Read the model definition and answer for the solid it produces. Units are mm, in the model's axes. Face numbers are marked on the shaded views. Coordinates: 2 decimals unless noted, no trailing zeros. Order: outer loops, then holes, each group sorted by start corner. A loop starts at its lowest first (then second) coordinate and runs counter-clockwise, first axis right, second up. Notation, with made-up numbers: M -0.5,88.25 L 50.5,88.25 A12 cw 50.5,101.25 Z; hole C 29,24 d1. An arc over 180 degrees is marked long. Put each result on its own line as item: value.
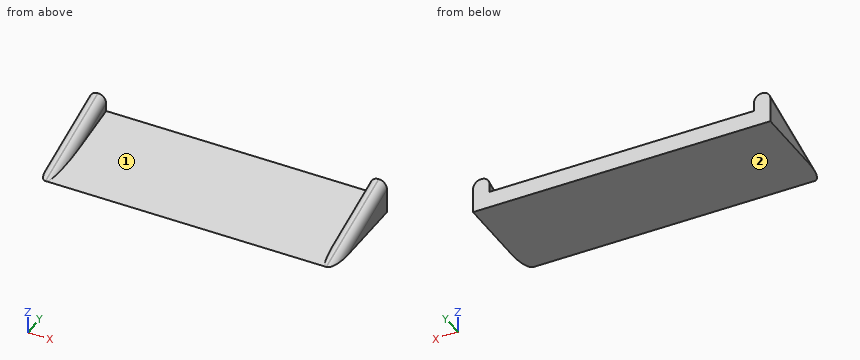
from build123d import *

# Parameters (mm, degrees)
F0_W     = 28.575
F0_H     = 9.525
F1_DEPTH = 1.5875
F3_DEPTH = 28.575
F5_DEPTH = 1.5875
F7_DEPTH = 1.5875
F8_R     = 0.762


with BuildPart() as f1:
    # F0 (on Top) → F1 (new body)
    with BuildSketch(Plane.XY):
        Rectangle(F0_W, F0_H)
    extrude(amount=F1_DEPTH)

    # F2 (on face) → F3 (cut, through all)
    with BuildSketch(Plane(origin=(-14.2875, 0, 0), x_dir=(0, -1, 0), z_dir=(-1, 0, 0))):
        Polygon((4.7625, 1.5875), (-4.7625, 1.5875), (4.7625, 0), align=None)
    extrude(amount=-F3_DEPTH, mode=Mode.SUBTRACT)

    # F4 (on face) → F5 (join)
    with BuildSketch(Plane(origin=(-14.2875, 0, 0), x_dir=(0, -1, 0), z_dir=(-1, 0, 0))):
        Polygon((-4.7625, 3.175), (-4.7625, 0), (4.7625, 0), align=None)
    extrude(amount=-F5_DEPTH)

    # F6 (on face) → F7 (join)
    with BuildSketch(Plane.YZ.offset(14.2875)):
        Polygon((-4.7625, 0), (4.7625, 0), (4.7625, 3.175), align=None)
    extrude(amount=-F7_DEPTH)

    # F8
    f8_edges = [f1.edges().sort_by_distance(p)[0] for p in [
        (-14.2875, 0, 1.5875),
        (-12.7, 0, 1.5875),
        (12.7, 0, 1.5875),
        (14.2875, 0, 1.5875),
    ]]
    fillet(f8_edges, radius=F8_R)


solid = f1.part
Q1. Given pin 1 (0.5 mm diameter, centred on y = 1, z = 1.5, fed in from +X); pin 2 (4 mm diameter, centred on x = -6.5, y = 0.5, fed in from +Z), each flat-ended and moving along its own axis, determine where each tip first touches the part or whether it passes through.
Answers below:
pin 1: stops at x = 14.28
pin 2: stops at z = 1.21
Q2. Find section A-A on x = -1.75. Write down the section's boundary in (y, z), plus the area to 3 significant figures.
Answers below:
outline: M -4.76,0 L 4.76,0 L 4.76,1.59 Z
area: 7.56 mm^2
Q3. Consider line 1 along Z through (x, y) = (5, 4.5); line 2 along Z through (x, y) = (-10, 0.5); line 3 along X through (y, z) = (-1, 0.95). Determine where each line is inside the solid, lowest interval first.
Answers below:
line 1: z = 0 to 1.54
line 2: z = 0 to 0.88
line 3: x = -14.12 to -12.86, 12.86 to 14.12
Q4. For a pull along X with two mould halves and no side action, classify the marked faces 1 and 2 as +X half, -X half, draft (parallel to the pull), parting line (faces both ways), or undercut.
Answers below:
face 1: undercut
face 2: draft
